Build history of the part. All positions in model axes, mm. A direction names the side the tool comes from. Round coordinates to 2 decimals unless told otherwise and drop trailing zeros. Order: outer loops, then holes, each group sorted by start corner. A loop starts at its lowest first (then second) coordinate and runs counter-clockwise, first axis right, second up. Notation, with made-up numbers: (3, 1.25) -> (11, 1.25) arc R38 ccw to (11, 39.25) -> close; hole circle Ø8 at (77.5, 21). An arc over 180 degrees is marked (long way). Use a Markdown table: item, result. Add a question column.
Item 1: Slice it at C-C, the plane z = 18. Give the cut face in (x, y).
Item 2: Slice it at A-A, the plane y = -30.5. Give the cut face in (x, z), plus the area to 3 significant figures.
Item 3: Two-plate mould, pull along Z, no slides. Class faces 1 (the face through (-88, -40, 70)), 2 (the face through (90, -7, 65)), 3 (the face through (-1, -6, -82.5)): released by +Z, released by -Z, zero draft, split by the parting line, or undercut.
Item 4: Slice it at B-B, the plane x = 15. Give the cut face in (y, z), plus the area to 3 significant figures.
Item 5: 3-axis set-ups, long thin cutter, end or side, ignore diameter. For faces 4 (the face through (75, -25, 70)), 5 (the face through (-1, -10, -1)), 6 (the face through (-90, -15, 70)), 7 (the face through (90, -7, 75)): which of +Z, -Z, +X, -X, +Y, -Y reach the whole face in a straight line?
Item 6: Probe L1, parallel to Y at x = -85, z = -78; L2, parallel to Z at x = -87, y = -5; L3, parallel to Z at x = 86.5, y = -33.5. List the from-to ranges inside material, lowest first.
Item 7: Pin check, flat tips, straight feed: pin 1 (1.5 mm diameter, centred on x = 94.5, y = -2.5, fed in from -Z); pin 2 (0.9 mm diameter, centred on x = 94.5, y = -2.5, fed in from +Z); pin 3 (5 mm diameter, centred on y = -5, z = -69, fed in from -X). Stop position of each tip, or through.
from build123d import *

# Parameters (mm, degrees)
SKETCH_3_W               = 200
SKETCH_3_H               = 165
EXTRUDE_1_DEPTH          = 10
SKETCH_4_W               = 25
SKETCH_4_H               = 25
EXTRUDE_2_DEPTH          = 30
SKETCH_5_W               = 20
SKETCH_5_H               = 10
CUT_EXTRUDE_2_DEPTH      = 15
MIRROR_2_COPY_1_SKETCH_W = 20
MIRROR_2_COPY_1_SKETCH_H = 10
MIRROR_2_COPY_1_DEPTH    = 15
SKETCH_6_R               = 1.5
CUT_EXTRUDE_3_DEPTH      = 20
MIRROR_4_COPY_1_SKETCH_R = 1.5
MIRROR_4_COPY_1_DEPTH    = 20


with BuildPart() as part:
    # 草图3 → 凸台-拉伸1 (new body)
    with BuildSketch(Plane(origin=(0, 0, 0), x_dir=(1, 0, 0), z_dir=(0, 1, 0))):
        Rectangle(SKETCH_3_W, SKETCH_3_H)
    extrude(amount=-EXTRUDE_1_DEPTH)

    # 草图4 → 凸台-拉伸2 (add)
    with BuildSketch(Plane.XZ.offset(10)):
        with Locations((-87.5, 70)):
            Rectangle(SKETCH_4_W, SKETCH_4_H)
        with Locations((87.5, 70)):
            Rectangle(SKETCH_4_W, SKETCH_4_H)
        with Locations((-87.5, -70)):
            Rectangle(SKETCH_4_W, SKETCH_4_H)
        with Locations((87.5, -70)):
            Rectangle(SKETCH_4_W, SKETCH_4_H)
    extrude(amount=EXTRUDE_2_DEPTH)

    # 草图5 → 切除-拉伸2 (cut)
    with BuildSketch(Plane(origin=(0, 0, 0), x_dir=(1, 0, 0), z_dir=(0, 1, 0))):
        with Locations((-90, 70)):
            Rectangle(SKETCH_5_W, SKETCH_5_H)
    cut_extrude_2 = extrude(amount=-CUT_EXTRUDE_2_DEPTH, mode=Mode.SUBTRACT)

    # 镜向1: 切除-拉伸2 across plane
    add(cut_extrude_2.mirror(Plane.XY), mode=Mode.SUBTRACT)

    # 镜向2: 切除-拉伸2 across plane
    add(cut_extrude_2.mirror(Plane(origin=(0, 0, 0), x_dir=(0, 0, 1), z_dir=(1, 0, 0))), mode=Mode.SUBTRACT)

    # 镜向2 copy 1 sketch → 镜向2 copy 1 (cut)
    with BuildSketch(Plane(origin=(0, 0, 0), x_dir=(-1, 0, 0), z_dir=(0, 1, 0))):
        with Locations((-90, 70)):
            Rectangle(MIRROR_2_COPY_1_SKETCH_W, MIRROR_2_COPY_1_SKETCH_H)
    extrude(amount=-MIRROR_2_COPY_1_DEPTH, mode=Mode.SUBTRACT)

    # 草图6 → 切除-拉伸3 (cut)
    with BuildSketch(Plane.XY.offset(82.5)):
        with Locations((-95, -3)):
            Circle(SKETCH_6_R)
        with Locations((-85, -3)):
            Circle(SKETCH_6_R)
        with Locations((-95, -12)):
            Circle(SKETCH_6_R)
        with Locations((-85, -12)):
            Circle(SKETCH_6_R)
    cut_extrude_3 = extrude(amount=-CUT_EXTRUDE_3_DEPTH, mode=Mode.SUBTRACT)

    # 镜向3: 切除-拉伸3 across plane
    add(cut_extrude_3.mirror(Plane.XY), mode=Mode.SUBTRACT)

    # 镜向4: 切除-拉伸3 across plane
    add(cut_extrude_3.mirror(Plane(origin=(0, 0, 0), x_dir=(0, 0, 1), z_dir=(1, 0, 0))), mode=Mode.SUBTRACT)

    # 镜向4 copy 1 sketch → 镜向4 copy 1 (cut)
    with BuildSketch(Plane(origin=(0, 0, -82.5), x_dir=(-1, 0, 0), z_dir=(0, 0, -1))):
        with Locations((-95, -3)):
            Circle(MIRROR_4_COPY_1_SKETCH_R)
        with Locations((-85, -3)):
            Circle(MIRROR_4_COPY_1_SKETCH_R)
        with Locations((-95, -12)):
            Circle(MIRROR_4_COPY_1_SKETCH_R)
        with Locations((-85, -12)):
            Circle(MIRROR_4_COPY_1_SKETCH_R)
    extrude(amount=-MIRROR_4_COPY_1_DEPTH, mode=Mode.SUBTRACT)


solid = part.part
Check sheet entries:
| question | item | result |
|---|---|---|
| 1 | outline | (-100, -10) -> (100, -10) -> (100, 0) -> (-100, 0) -> close |
| 2 | outline | (-100, -82.5) -> (-75, -82.5) -> (-75, -57.5) -> (-100, -57.5) -> close; (-100, 57.5) -> (-75, 57.5) -> (-75, 82.5) -> (-100, 82.5) -> close; (75, -82.5) -> (100, -82.5) -> (100, -57.5) -> (75, -57.5) -> close; (75, 57.5) -> (100, 57.5) -> (100, 82.5) -> (75, 82.5) -> close |
| 2 | area | 2,500 mm2 |
| 3 | face 1 | zero draft |
| 3 | face 2 | undercut |
| 3 | face 3 | released by -Z |
| 4 | outline | (-10, -82.5) -> (0, -82.5) -> (0, 82.5) -> (-10, 82.5) -> close |
| 4 | area | 1,650 mm2 |
| 5 | face 4 | +Z, -Z, -Y |
| 5 | face 5 | -Y |
| 5 | face 6 | -X, +Y |
| 5 | face 7 | +X, +Y |
| 6 | L1 | -40 to -13.5, -10.5 to -4.5, -1.5 to 0 |
| 6 | L2 | -82.5 to -75, -65 to 65, 75 to 82.5 |
| 6 | L3 | -82.5 to -57.5, 57.5 to 82.5 |
| 7 | pin 1 | z = -62.5 |
| 7 | pin 2 | z = 62.5 |
| 7 | pin 3 | x = -80 |
